Verification items for the finished model (mm, model axes). Round coordinates to 2 decimals unless told otherwise and drop trailing zeros. Write each loop counter-clockwise with the first axis right and the second up, starting at its lowest first coordinate (ties: lowest second). Pieces come first, ordered by that corner, then holes.
from build123d import *

# Parameters (mm, degrees)
BOSS_EXTRUDE1_DEPTH = 1
SKETCH2_R           = 3.175
CUT_EXTRUDE1_DEPTH  = 2
SKETCH3_W           = 2.54
SKETCH3_H           = 0.635
CUT_EXTRUDE2_DEPTH  = 2


with BuildPart() as part:
    # Sketch1 → Boss-Extrude1 (new body)
    with BuildSketch(Plane.XY):
        with BuildLine():
            Line((67.21146711, 76.191723231), (8.696654013, 17.676910134))
            Line((8.696654013, 17.676910134), (7.228954972, 14.133571205))
            ThreePointArc((7.228954972, 14.133571205), (14.666587579, 6.075099489), (15.105587123, -4.88230096))
            Line((15.105587123, -4.88230096), (18.648926052, -6.35))
            Line((18.648926052, -6.35), (101.401368334, -6.35))
            ThreePointArc((101.401368334, -6.35), (93.866160503, 38.880636728), (67.21146711, 76.191723231))
        make_face()
        with BuildLine():
            Line((88.672924278, 6.35), (27.86051193, 6.35))
            ThreePointArc((27.86051193, 6.35), (26.399857642, 10.93517908), (24.190484974, 15.210228852))
            Line((24.190484974, 15.210228852), (67.191354125, 58.211098004))
            ThreePointArc((67.191354125, 58.211098004), (82.13289044, 34.020557137), (88.672924278, 6.35))
        make_face(mode=Mode.SUBTRACT)
    extrude(amount=BOSS_EXTRUDE1_DEPTH)

    # Sketch2 → Cut-Extrude1 (cut, through all)
    with BuildSketch(Plane.XY.offset(1)):
        with Locations((22.225, 0)):
            Circle(SKETCH2_R)
        with Locations((36.195, 0)):
            Circle(SKETCH2_R)
        with Locations((61.722, 0)):
            Circle(SKETCH2_R)
        with Locations((75.692, 0)):
            Circle(SKETCH2_R)
        with Locations((95.25, 0)):
            Circle(SKETCH2_R)
        with Locations((15.715448212, 15.715448212)):
            Circle(SKETCH2_R)
        with Locations((25.593729945, 25.593729945)):
            Circle(SKETCH2_R)
        with Locations((43.644044748, 43.644044748)):
            Circle(SKETCH2_R)
        with Locations((53.522326482, 53.522326482)):
            Circle(SKETCH2_R)
        with Locations((92.004434954, 24.652514046)):
            Circle(SKETCH2_R)
        with Locations((82.48891971, 47.625)):
            Circle(SKETCH2_R)
        with Locations((67.351920908, 67.351920908)):
            Circle(SKETCH2_R)
    extrude(amount=-CUT_EXTRUDE1_DEPTH, mode=Mode.SUBTRACT)

    # Sketch3 → Cut-Extrude2 (cut, through all)
    with BuildSketch(Plane.XY.offset(1)):
        Polygon((15.266435406, 24.246691527), (17.06248663, 26.042742751), (17.511499436, 25.593729945), (15.715448212, 23.797678721), align=None)
        Polygon((44.991083167, 53.971339288), (43.195031942, 52.175288063), (43.644044748, 51.726275257), (45.440095973, 53.522326482), align=None)
        with Locations((29.21, -6.0325)):
            Rectangle(SKETCH3_W, SKETCH3_H)
        with Locations((68.707, -6.0325)):
            Rectangle(SKETCH3_W, SKETCH3_H)
        Polygon((29.230733674, 38.210989795), (31.026784898, 40.007041019), (31.475797704, 39.558028213), (29.67974648, 37.761976989), align=None)
        Polygon((56.845021246, 65.825277367), (55.048970022, 64.029226143), (55.497982828, 63.580213337), (57.294034052, 65.376264561), align=None)
        with Locations((48.9585, -6.0325)):
            Rectangle(SKETCH3_W, SKETCH3_H)
        with Locations((85.471, -6.0325)):
            Rectangle(SKETCH3_W, SKETCH3_H)
        Polygon((99.935462164, 14.437711971), (100.266998693, 11.919442024), (101.526133667, 12.085210288), (101.194597138, 14.603480236), align=None)
        Polygon((93.765504959, 37.464305742), (94.938831965, 37.950313702), (93.966816047, 40.296967714), (92.793489041, 39.810959755), align=None)
        Polygon((79.327792988, 62.471156422), (80.874047017, 60.456038938), (81.88160576, 61.229165953), (80.33535173, 63.244283437), align=None)
        Polygon((13.979268531, 4.415764523), (28.059192607, 10.247860033), (27.087176689, 12.594514045), (13.007252613, 6.762418536), align=None)
    extrude(amount=-CUT_EXTRUDE2_DEPTH, mode=Mode.SUBTRACT)


solid = part.part
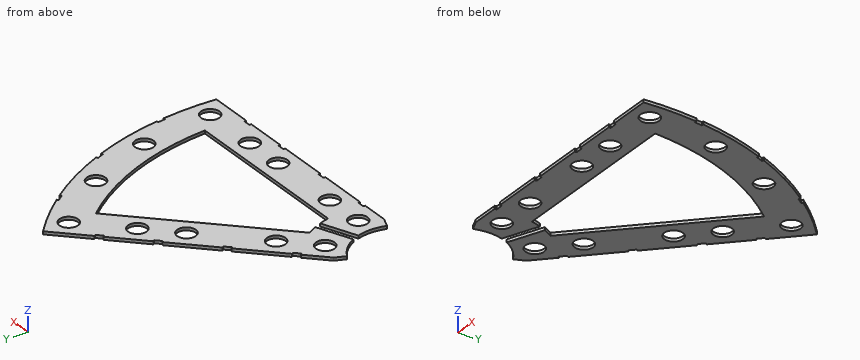
Q1. Sectioned sample at C-C (y = 69). Enter the section's corners in (x, z), plus the area to 3 significant figures.
Recorded:
outline: (60.02, 0) - (64.64, 0) - (64.64, 1) - (60.02, 1) - close; (70.07, 0) - (74.58, 0) - (74.58, 1) - (70.07, 1) - close
area: 9.13 mm2
Q2. Sectioned sample at B-B (x = 37.5). Enter the section's corners in (y, z).
Recorded:
outline: (-6.35, 0) - (-2.89, 0) - (-2.89, 1) - (-6.35, 1) - close; (2.89, 0) - (6.35, 0) - (6.35, 1) - (2.89, 1) - close; (28.52, 0) - (46.48, 0) - (46.48, 1) - (28.52, 1) - close
Q3. Sectioned sample at A-A (y = 0). Enter the section's corners in (x, z) (3 decimals).
Recorded:
outline: (15.875, 0) - (19.05, 0) - (19.05, 1) - (15.875, 1) - close; (25.4, 0) - (33.02, 0) - (33.02, 1) - (25.4, 1) - close; (39.37, 0) - (58.547, 0) - (58.547, 1) - (39.37, 1) - close; (64.897, 0) - (72.517, 0) - (72.517, 1) - (64.897, 1) - close; (78.867, 0) - (92.075, 0) - (92.075, 1) - (78.867, 1) - close; (98.425, 0) - (101.6, 0) - (101.6, 1) - (98.425, 1) - close
Q4. Sectioned sample at D-D (z = 0.25). Give the number of separate pieces and of enclosed holes in the cut face, plus the area to 3 significant figures.
Recorded:
separate pieces: 1
enclosed holes: 12
area: 2,600 mm2
Q5. Material ranges on line 1 along Y through (x, z) = (16, 0.9); line 2 along Y through (x, z) = (74.5, 0.9); line 3 along X through (y, z) = (42, 0.2), recorded low to high.
Recorded:
line 1: y = -5.25 to 5.25, 8 to 12.55, 18.88 to 24.08
line 2: y = -6.35 to -2.94, 2.94 to 6.35, 48.51 to 69.08
line 3: x = 33.02 to 40.93, 46.36 to 50.98, 78.35 to 92.51
Q6. Depth check by flat-ended pin: P1, Ø6, axis at x = 77, y = 38, coming from the +Z side; P2, Ø0.5, axis at x = 29.5, z = 0.5, coming from the -Y side (3 decimals). Enter the tip coordinate at first touch or a pass-through.
Recorded:
P1: passes through
P2: stops at y = -5.715
